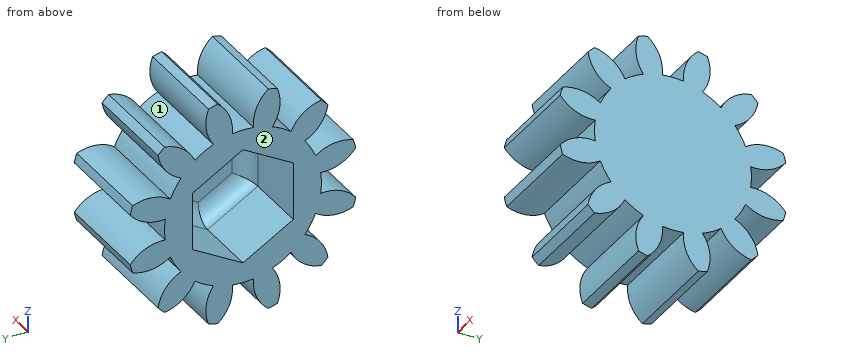
from build123d import *

# Parameters (mm, degrees)
BASPROSKE_W         = 9.525
BASPROSKE_H         = 11.1125
TOOTHCUT_DEPTH      = 19.376641083
TEETHCUTS_COUNT     = 12
BORSKE_R            = 3.175
BORE_DEPTH          = 9.525
BOSS_EXTRUDE1_START = -25.4
SKETCH2_R           = 7.539355
BOSS_EXTRUDE1_DEPTH = 25.4
CUT_EXTRUDE1_DEPTH  = 20
SKETCH5_R           = 1.905
CUT_EXTRUDE2_DEPTH  = 24.605363577
SKETCH6_R           = 12.7
SKETCH6_R_2         = 5.7785
CUT_EXTRUDE3_DEPTH  = 15.875
SKETCH7_R           = 5.7785
CUT_EXTRUDE4_DEPTH  = 23.070094739
BOSS_EXTRUDE2_START = 4.125
BOSS_EXTRUDE2_DEPTH = 4.125
CUT_EXTRUDE5_DEPTH  = 7.62
FILLET1_R           = 1.5875


with BuildPart() as part:
    # BasProSke → Base-Revolve (revolve)
    with BuildSketch(Plane(origin=(0, 0, 0), x_dir=(1, 0, 0), z_dir=(0, 1, 0)), mode=Mode.PRIVATE) as base_revolve_sk:
        with Locations((4.7625, 5.55625)):
            Rectangle(BASPROSKE_W, BASPROSKE_H)
    revolve(base_revolve_sk.sketch.rotate(Axis((-10, 0, 0), (1, 0, 0)), 180), axis=Axis((-10, 0, 0), (1, 0, 0)))

    # TooCutSke → ToothCut (cut, through all)
    with BuildSketch(Plane(origin=(0, 0, 0), x_dir=(0, 0, -1), z_dir=(1, 0, 0))):
        with BuildLine():
            ThreePointArc((1.026937745, 7.469087808), (0, 7.539355), (-1.026937745, 7.469087808))
            ThreePointArc((-1.026937745, 7.469087808), (-1.30857978, 9.35080814), (-2.465050847, 10.861691431))
            ThreePointArc((-2.465050847, 10.861691431), (0, 11.1379), (2.465050847, 10.861691431))
            ThreePointArc((2.465050847, 10.861691431), (1.30857978, 9.35080814), (1.026937745, 7.469087808))
        make_face()
    toothcut = extrude(amount=TOOTHCUT_DEPTH, mode=Mode.SUBTRACT)

    # TeethCuts: ToothCut ×12 about axis
    teethcuts_axis = Axis((0, 0, 0), (1, 0, 0))
    for i in range(1, TEETHCUTS_COUNT):
        add(toothcut.rotate(teethcuts_axis, i * 360 / TEETHCUTS_COUNT), mode=Mode.SUBTRACT)

    # BorSke → Bore (cut, symmetric)
    with BuildSketch(Plane(origin=(0, 0, 0), x_dir=(0, 0, -1), z_dir=(1, 0, 0))):
        with Locations(Location((0, 0, 0), (0, 0, 180))):
            Circle(BORSKE_R)
    extrude(amount=BORE_DEPTH, both=True, mode=Mode.SUBTRACT)

    # Sketch2 → Boss-Extrude1 (add)
    with BuildSketch(Plane(origin=(9.525, 0, 0), x_dir=(0, 0, -1), z_dir=(1, 0, 0)).offset(BOSS_EXTRUDE1_START)):
        with Locations(Location((0, 0, 0), (0, 0, 172.171388978))):
            Circle(SKETCH2_R)
    extrude(amount=BOSS_EXTRUDE1_DEPTH)

    # Sketch3 → Cut-Extrude1 (cut)
    with BuildSketch(Plane.ZY.offset(15.875)):
        with BuildLine():
            Line((-1.778, 2.8575), (1.778, 2.8575))
            ThreePointArc((1.778, 2.8575), (0, -3.3655), (-1.778, 2.8575))
        make_face()
    extrude(amount=-CUT_EXTRUDE1_DEPTH, mode=Mode.SUBTRACT)

    # Sketch5 → Cut-Extrude2 (cut, through all)
    with BuildSketch(Plane.XZ.offset(-2.8575)):
        with Locations(Location((-12.065, 0, 0), (0, 0, 270))):
            Circle(SKETCH5_R)
    extrude(amount=-CUT_EXTRUDE2_DEPTH, mode=Mode.SUBTRACT)

    # Sketch6 → Cut-Extrude3 (cut)
    with BuildSketch(Plane.ZY.offset(15.875)):
        Circle(SKETCH6_R)
        Circle(SKETCH6_R_2, mode=Mode.SUBTRACT)
    extrude(amount=-CUT_EXTRUDE3_DEPTH, mode=Mode.SUBTRACT)

    # Sketch7 → Cut-Extrude4 (cut, through all)
    with BuildSketch(Plane.ZY):
        Circle(SKETCH7_R)
    extrude(amount=CUT_EXTRUDE4_DEPTH, mode=Mode.SUBTRACT)

    # Sketch8 → Boss-Extrude2 (add)
    with BuildSketch(Plane.ZY.offset(-4.125).offset(BOSS_EXTRUDE2_START)):
        with BuildLine():
            Line((1.778, 2.8575), (-1.778, 2.8575))
            ThreePointArc((-1.778, 2.8575), (0, -3.3655), (1.778, 2.8575))
        make_face()
    extrude(amount=-BOSS_EXTRUDE2_DEPTH)

    # Sketch9 → Cut-Extrude5 (cut)
    with BuildSketch(Plane.ZY):
        Polygon((5.588, 0), (2.794, 4.839349956), (-2.794, 4.839349956), (-5.588, 0), (-2.794, -4.839349956), (2.794, -4.839349956), align=None)
    extrude(amount=-CUT_EXTRUDE5_DEPTH, mode=Mode.SUBTRACT)

    # Fillet1
    fillet1_edges = [part.edges().sort_by_distance(p)[0] for p in [
        (7.62, 4.839349956, 0),
        (7.62, 2.419674978, 4.191),
        (7.62, -2.419674978, 4.191),
        (7.62, -4.839349956, 0),
        (7.62, -2.419674978, -4.191),
        (7.62, 2.419674978, -4.191),
    ]]
    fillet(fillet1_edges, radius=FILLET1_R)


solid = part.part
Could you check a few things on this model? Use its own coordinates, in mm. Face numbers are marked on the shaded views. Round coordinates to 2 decimals unless told otherwise and drop trailing zeros. Order: outer loops, then holes, each group sorted by start corner. A loop starts at its lowest first (then second) coordinate and runs counter-clockwise, first axis right, second up.
(1) Imagine slicing it at B-B (z = -1.5). Write out the boundary of the cut face in (x, y) (1 decimal), plus the area to 3 significant figures.
Response values:
outline: (0, -9.7) - (9.5, -9.7) - (9.5, 9.7) - (0, 9.7) - (0, 4.8) - (6, 4.8) arc R1.6 cw to (7.6, 3.3) - (7.6, -3.3) arc R1.6 cw to (6, -4.8) - (0, -4.8) - close
area: 113 mm2
(2) I'm going to push flat-ended pins straight in: pin 1 (1 mm diameter, centred on x = 7.5, y = 1, fed in from +Z); pin 2 (3 mm diameter, centred on x = 6.5, z = 0, fed in from +Y); pin 3 (2 mm diameter, centred on y = 8, z = -3.5, fed in from +X) (3 decimals); pin 4 (5 mm diameter, centred on y = 0, z = -0.5, fed in from -X). Where does each tip first touch, or does it pass through?
Response values:
pin 1: stops at z = 9.74
pin 2: stops at y = 9.74
pin 3: stops at x = 9.525
pin 4: stops at x = 7.62
(3) If we mould it in two halves opening along Z, with no side actions, what happens to the marked faces 1 and 2? For each: released by +Z, released by -Z, zero draft, split by the parting line, or undercut.
Response values:
face 1: undercut
face 2: zero draft
(4) Please list where these lines run through material, in increasing order: line 1 along Y through (x, z) = (5.5, -0.25); line 2 along Y through (x, z) = (6.5, 7.25); line 3 along Y through (x, z) = (8.75, -6.5).
Response values:
line 1: y = -7.54 to -4.84, 4.84 to 7.54
line 2: y = -8.12 to -5.57, -3.02 to 3.02, 5.57 to 8.12
line 3: y = -7.86 to -4.92, -3.82 to 3.82, 4.92 to 7.86
(5) Imagine slicing it at C-C (y = 8.75). Write out the boundary of the cut face in (x, z) (3 decimals), plus the area to 3 significant figures.
Response values:
outline: (0, -3.542) - (9.525, -3.542) - (9.525, -1.111) - (0, -1.111) - close; (0, 1.111) - (9.525, 1.111) - (9.525, 3.542) - (0, 3.542) - close
area: 46.3 mm2
(6) Imagine slicing it at A-A (y = 6.25). Write out the boundary of the cut face in (x, z) (3 decimals).
Response values:
outline: (0, -7.731) - (9.525, -7.731) - (9.525, -4.771) - (0, -4.771) - close; (0, -4.217) - (9.525, -4.217) - (9.525, 4.217) - (0, 4.217) - close; (0, 4.771) - (9.525, 4.771) - (9.525, 7.731) - (0, 7.731) - close
